The listing builds one solid part. Answer for the finished solid, in the listing's coordinates (mm). Coordinates: 2 decimals unless noted, no trailing zeros. Write each loop counter-clockwise with the first axis right and the second up, starting at its lowest first coordinate (ties: lowest second). Pieces come first, ordered by that corner, then holes.
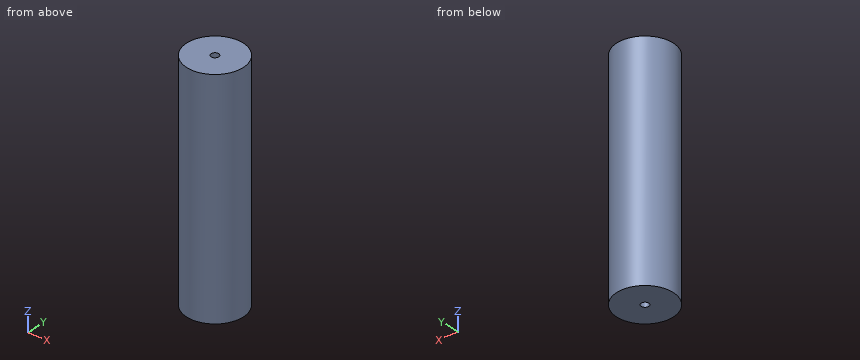
Autodesk Inventor part; units mm, degrees
ref_plane "YZ Plane" through (0, 0, 0) normal (1, 0, 0) x (0, 1, 0)
ref_plane "XZ Plane" through (0, 0, 0) normal (0, 1, 0) x (-1, 0, 0)
ref_plane "XY Plane" through (0, 0, 0) normal (0, 0, 1) x (1, 0, 0)
sketch "Sketch1" plane through (0, 0, 0) normal (0, 0, 1) x (1, 0, 0)
  circle A0 centre (0, 0) radius 9.525
  dimension "d0" = 19.05
extrude "Extrusion1" add sketch "Sketch1" along normal blind 76.2
sketch "Sketch2" plane through (0, 0, 76.2) normal (0, 0, 1) x (1, 0, 0)
  circle A0 centre (0, 0) radius 9.525
  circle A1 centre (0, 0) radius 1.27
  dimension "d3" = 2.54
extrude "Extrusion2" cut sketch "Sketch2" against normal blind 7.62 contours A1
sketch "Sketch3" plane through (0, 0, 0) normal (0, 0, -1) x (-1, 0, 0)
  circle A0 centre (0, 0) radius 9.525
  circle A1 centre (0, 0) radius 1.27
  circle A2 centre (0, 0) radius 1.27
hole "Hole1" at (0, 0, 0) direction (0, 0, 1) diameter 2.54 end through all
properties part number "Rod"
(1) Section A-A, the plane z = 44 is taken. Write down the section's boundary in (x, y) (3 decimals).
(2) Each of these flat-tipped pins is pushed along its axis until it touches: pin 1 (8 mm diameter, centred on x = 7, z = 33, fed in from -Y); pin 2 (4 mm diameter, centred on y = 7, z = 15, fed in from +X); pin 3 (10 mm diameter, centred on x = 5.5, z = 34.5, fed in from -Y). Where does it stop, or does it pass through?
(3) Section C-C, the plane x = -4.75 is taken. Write down the section's boundary in (y, z).
(4) Section B-B, the plane y = 2.5 is taken. Write down the section's boundary in (x, z).
(5) Find the intervals of material crossed by probe 1 along Y at (x, z) = (0, 35.5) (3 decimals); probe 2 along Y at (x, z) = (0.5, 72); probe 3 along Y at (x, z) = (-7.5, 45), in increasing order.
Solution:
1. outline: circle Ø19.05 at (0, 0); hole circle Ø2.54 at (0, 0)
2. pin 1: stops at y = -9.04
2. pin 2: stops at x = 8.11
2. pin 3: stops at y = -9.51
3. outline: (-8.26, 0) - (8.26, 0) - (8.26, 76.2) - (-8.26, 76.2) - close
4. outline: (-9.19, 0) - (9.19, 0) - (9.19, 76.2) - (-9.19, 76.2) - close
5. probe 1: y = -9.525 to -1.27, 1.27 to 9.525
5. probe 2: y = -9.51 to -1.17, 1.17 to 9.51
5. probe 3: y = -5.87 to 5.87
